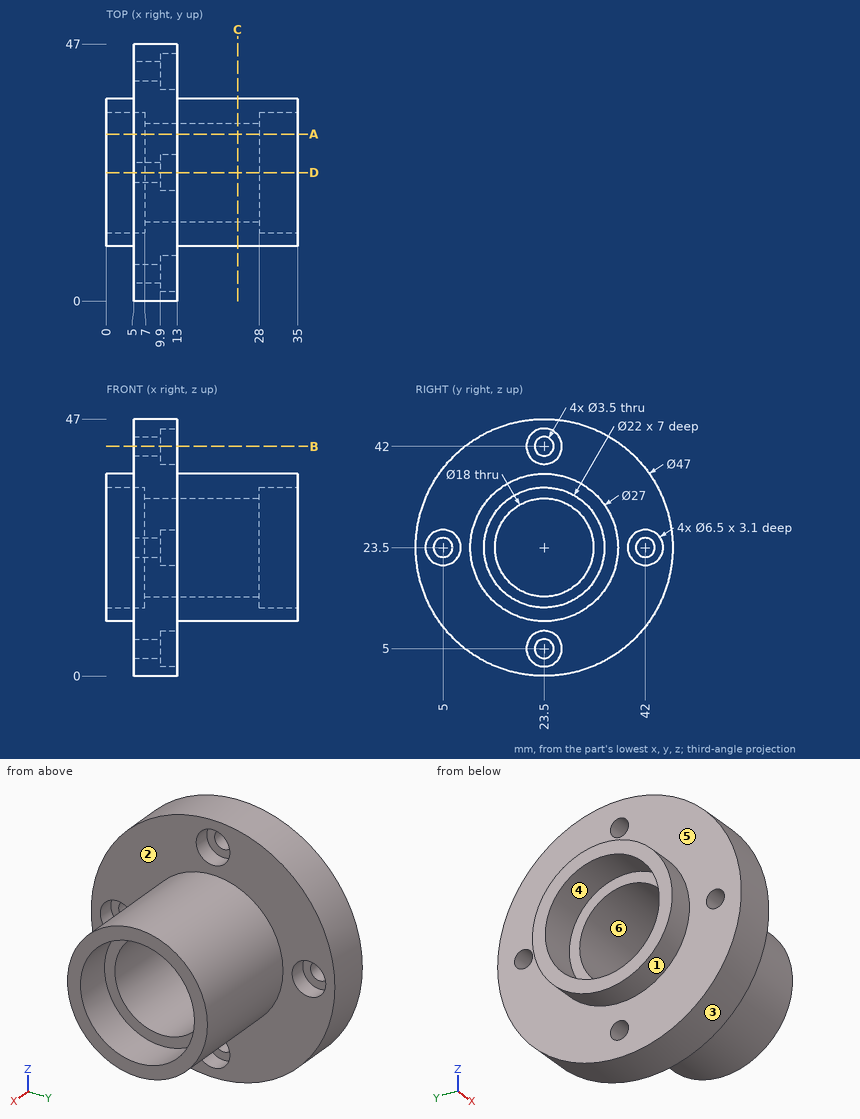
For this review, use the dimensioned drawing (mm, ordinates from the lowest corner) and the shaded views. A direction names the side the tool comes from. Give positions to 0.01 mm unless a question says otherwise; leave off trailing zeros. Order: outer loops, then holes, each group sorted by start corner. A loop starts at its lowest first (then second) coordinate and runs counter-clockwise, first axis right, second up.
1) Take a section at A-A (y = 30.5). Give the boundary of the cut face in (x, z), then the cut area to 3 significant figures.
2) Take a section at C-C (x = 24). Give the boundary of the cut face in (y, z), then the cut area to 3 significant figures.
3) Take a section at B-B (z = 42). Give the boundary of the cut face in (x, y), then the cut area to 3 significant figures.
4) The part is to be moulded in two halves that separate along Z. For the marked faces 3, 4, 5 and 6, say which applies: released by +Z, released by -Z, zero draft, split by the parting line, or undercut.
5) Wall thickness on line 1 (Z direction, x = 11.65, y = 23.5); line 2 (Z direction, x = 30, y = 24); line 3 (Y direction, x = 31.5, z = 23.5): over which ranges is each line inside the solid? List them lowest first.
6) Insertion check: pin 1 (8.5 mm diameter, centred on y = 5, z = 23.5, fed in from -X); pin 2 (7 mm diameter, centred on y = 22, z = 6.5, fed in from +X); pin 3 (6.5 mm diameter, centred on y = 22.5, z = 27, fed in from +X); pin 4 (3 mm diameter, centred on x = 28.5, y = 18, fed in from -Z). Each pin has a flat end and moves straight along its axis. Give the tip position at first contact, or say it passes through.
7) For the marked faces 1 and 2, list the 3-axis set-ups (+Z, -Z, +X, -X, +Y, -Y) from which the entire face can be reached by the end or side of a thin tool; tool diameter is ignored.
8) Take a section at D-D (y = 23.5). State how many separate pieces and enclosed holes the cut face has, then the cut area to 3 significant figures.
Derived:
1. outline: (0, 11.96) - (5, 11.96) - (5, 1.07) - (13, 1.07) - (13, 11.96) - (35, 11.96) - (35, 15.01) - (28, 15.01) - (28, 17.84) - (7, 17.84) - (7, 15.01) - (0, 15.01) - close; (0, 31.99) - (7, 31.99) - (7, 29.16) - (28, 29.16) - (28, 31.99) - (35, 31.99) - (35, 35.04) - (13, 35.04) - (13, 45.93) - (5, 45.93) - (5, 35.04) - (0, 35.04) - close
1. area: 507 mm2
2. outline: circle Ø27 at (23.5, 23.5); hole circle Ø18 at (23.5, 23.5)
2. area: 318 mm2
3. outline: (5, 9.01) - (13, 9.01) - (13, 20.25) - (9.9, 20.25) - (9.9, 21.75) - (5, 21.75) - close; (5, 25.25) - (9.9, 25.25) - (9.9, 26.75) - (13, 26.75) - (13, 37.99) - (5, 37.99) - close
3. area: 195 mm2
4. face 3: split by the parting line
4. face 4: undercut
4. face 5: zero draft
4. face 6: undercut
5. line 1: z = 0 to 1.75, 8.25 to 14.5, 32.5 to 38.75, 45.25 to 47
5. line 2: z = 10.01 to 12.51, 34.49 to 36.99
5. line 3: y = 10 to 12.5, 34.5 to 37
6. pin 1: stops at x = 5
6. pin 2: stops at x = 13
6. pin 3: passes through
6. pin 4: stops at z = 10.61
7. face 1: -X
7. face 2: +X
8. separate pieces: 4
8. enclosed holes: 0
8. area: 344 mm2
